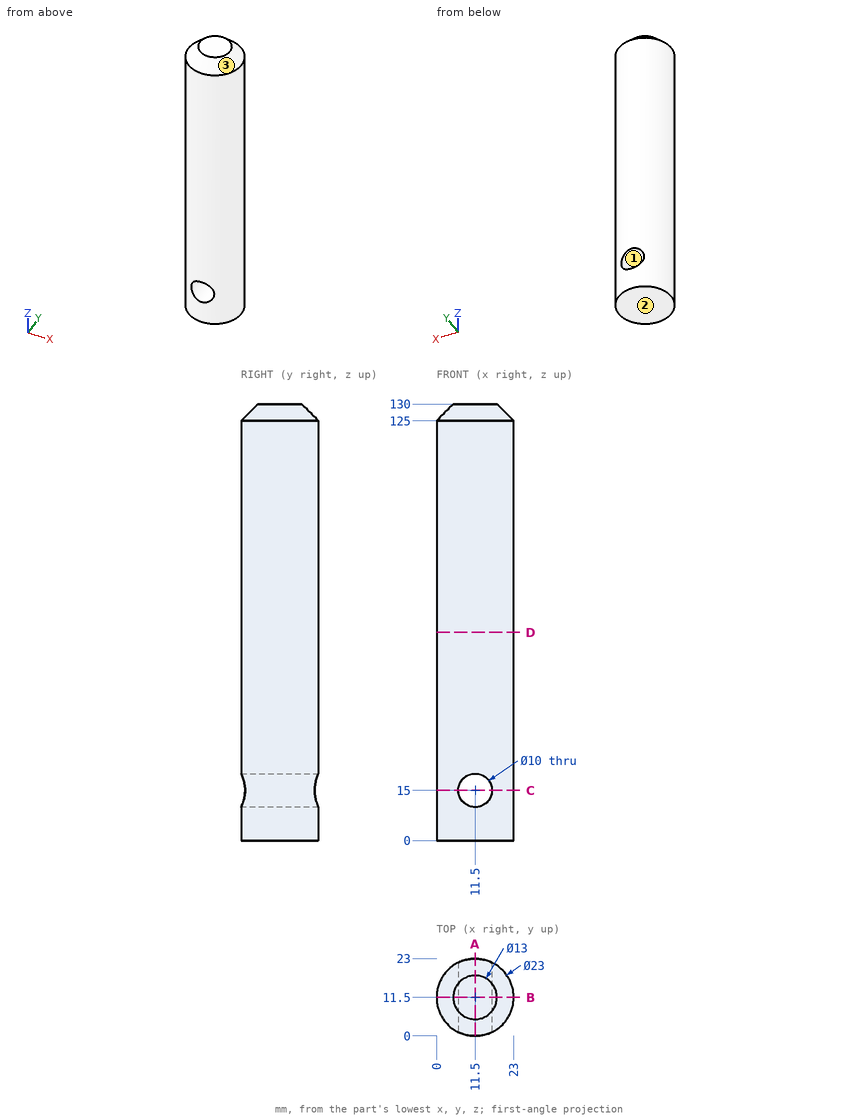
Here's the drawing with two shaded views (mm, measured from the low corner). I have some questions. Give positions to 0.01 mm unless a question says otherwise; leave off trailing zeros. Order: outer loops, then holes, each group sorted by start corner. A loop starts at its lowest first (then second) coordinate and runs counter-clockwise, first axis right, second up.
Q1. Suppose I cut it at A-A, the plane x = 11.5. Write out the boundary of the cut face in (y, z), and give its area (4 significant figures).
Q2. We'd pull the mould along X, two halves only. Please class the marked faces 1, 2 and 3: +X half, -X half, draft (parallel to the pull), parting line (faces both ways), or undercut.
Q3. Suppose I cut it at D-D, the plane z = 62. Write out the boundary of the cut face in (x, y), and give its area (3 significant figures).
Q4. Suppose I cut it at B-B, the plane y = 11.5. Write out the boundary of the cut face in (x, z), and give its area (3 significant figures).
Q5. Suppose I cut it at C-C, the plane z = 15. Write out the boundary of the cut face in (x, y), and give its area (3 significant figures).
Q6. I'm going to push flat-ended pins straight in: P1, Ø2, axis at x = 6.5, z = 81, coming from the +Y side; P2, Ø1, axis at x = 6.5, z = 98, coming from the +Y side; P3, Ø6, axis at x = 3, y = 4.5, coming from the +Z side. Where does each tip first touch, or does it pass through?
Q7. If I drill on line 1 along X through (y, z) = (11.75, 15); line 2 along Z through (x, y) = (11, 16); line 3 along Z through (x, y) = (15, 10.5), over which ranges is the centre line in solid material (lowest first)?
Solution:
1. outline: (0, 0) - (23, 0) - (23, 10) - (0, 10) - close; (0, 20) - (23, 20) - (23, 125) - (18, 130) - (5, 130) - (0, 125) - close
1. area: 2,735 mm2
2. face 1: undercut
2. face 2: draft
2. face 3: parting line
3. outline: circle Ø23 at (11.5, 11.5)
3. area: 415 mm2
4. outline: (0, 0) - (23, 0) - (23, 125) - (18, 130) - (5, 130) - (0, 125) - close; hole circle Ø10 at (11.5, 15)
4. area: 2,890 mm2
5. outline: (6.5, 1.14) - (6.5, 21.86) arc R11.5 ccw to start; (16.5, 1.14) arc R11.5 ccw to (16.5, 21.86) - close
5. area: 193 mm2
6. P1: stops at y = 22.28
6. P2: stops at y = 22.08
6. P3: stops at z = 128.49
7. line 1: x = 0 to 6.5, 16.5 to 23
7. line 2: z = 0 to 10.03, 19.97 to 130
7. line 3: z = 0 to 11.43, 18.57 to 130
